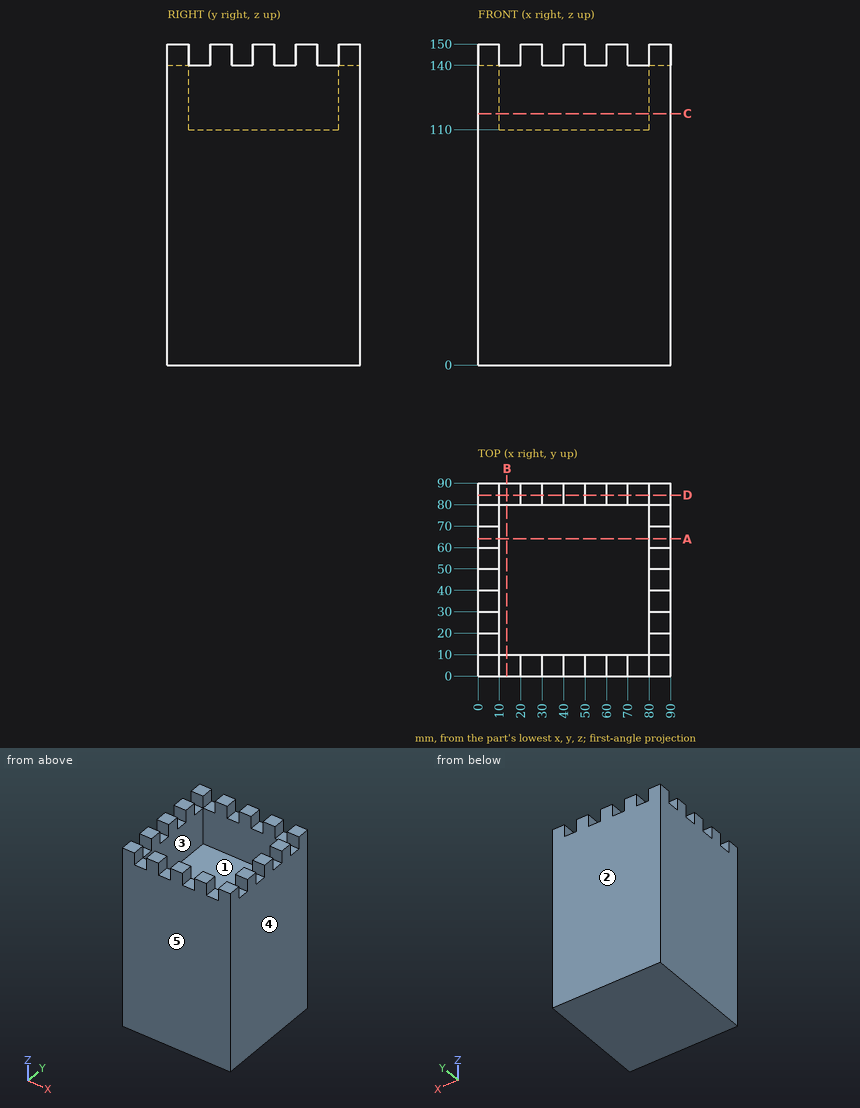
Input: dimensioned drawing with shaded views. Units: mm. Origin: part minimum x, y, z. A direction names the side the tool comes from. Give positions to 0.01 mm unless a question says otherwise; leave off trailing zeros. Loops run counter-clockwise (first coordinate to the right, second up) from the corner with the lowest first, then second, coordinate; pieces in that order, holes last. Notation, with made-up numbers: M 28.5,18 L 68.5,18 A26 cw 68.5,32 Z; hole C 14.25,74 d4. An arc over 180 degrees is marked long. Put each result on its own line as item: value.
1) Reachability of the marked faces 1 and 2 from +Z, -Z, +X, -X, +Y, -Y: full face, straight path, thin tool, end or side. Return the list, or none.
Computed values:
face 1: +Z
face 2: +Z, -Z, +X, -X, +Y
2) Cut plane C-C, the plane z = 117.5. Return the cut outline in (x, y), plus the area to 3 significant figures.
Computed values:
outline: M 0,0 L 90,0 L 90,90 L 0,90 Z; hole M 10,10 L 80,10 L 80,80 L 10,80 Z
area: 3,200 mm^2
3) Mould query, pull axis X, two halves, no side actions, for the marked faces 3, 4 and 5. Classes: released by +X, released by -X, zero draft, split by the parting line, or undercut.
Computed values:
face 3: undercut
face 4: released by +X
face 5: zero draft
4) First-contact query: P1, Ø3, axis at y = 83.5, z = 146, coming from the -X side; P2, Ø10, axis at x = 57, y = 32, coming from the +Z side; P3, Ø3, axis at x = 17.5, y = 85, coming from the +Z side. Flat tips, straight axial feed; report the tip coordinate or a pass-through.
Computed values:
P1: stops at x = 0
P2: stops at z = 110
P3: stops at z = 140
5) Cut plane B-B, the plane x = 13.5. Return the cut outline in (y, z), plus the area to 3 significant figures.
Computed values:
outline: M 0,0 L 90,0 L 90,140 L 80,140 L 80,110 L 10,110 L 10,140 L 0,140 Z
area: 10,500 mm^2
6) Material intervals for L1, parallel to Y at x = 77, z = 136.5; L2, parallel to Z at x = 65, y = 60.5, sorted ascending. Write a range as from..to.
Computed values:
L1: y = 0..10, 80..90
L2: z = 0..110
7) Cut plane A-A, the plane y = 64. Return the cut outline in (x, z), plus the area to 3 significant figures.
Computed values:
outline: M 0,0 L 90,0 L 90,150 L 80,150 L 80,110 L 10,110 L 10,150 L 0,150 Z
area: 10,700 mm^2
8) Cut plane D-D, the plane y = 84.5. Return the cut outline in (x, z), plus the area to 3 significant figures.
Computed values:
outline: M 0,0 L 90,0 L 90,150 L 80,150 L 80,140 L 70,140 L 70,150 L 60,150 L 60,140 L 50,140 L 50,150 L 40,150 L 40,140 L 30,140 L 30,150 L 20,150 L 20,140 L 10,140 L 10,150 L 0,150 Z
area: 13,100 mm^2
